Verification items for the finished model (mm, model axes). Face numbers are marked on the shaded views. A direction names the side the tool comes from. Coordinates: 2 decimals unless noted, no trailing zeros. Write each loop counter-clockwise with the first axis right and the second up, starting at its lowest first coordinate (ties: lowest second). Pieces come first, ordered by that corner, then holes. Notation, with made-up numbers: (-2.5, 65.5) -> (47.5, 65.5) arc R21 cw to (47.5, 90.5) -> close; hole circle Ø8 at (87.5, 44.5). An arc over 180 degrees is marked (long way). Write item = value, one per line. Start each with the question number.
(1) Set-up check for the marked faces 1, 2 and 3: record each of +Z, -Z, +X, -X, +Y, -Y from which the full face is reachable in a straight line by a thin tool's end or side.
(2) Material ranges on probe 1 along Z at (x, y) = (16, 57); probe 2 along Y at (x, z) = (-27, -1); probe 3 along X at (y, z) = (105, -10.5), recorded low to high. Write a range as [from, to].
(3) Section check A-A (y = 48.5). Record the cut outline in (x, z).
(4) Section check C-C (z = 8). Record the cut outline in (x, y), plus the area to 3 significant figures.
(5) Gauge pin test, flat ends, axial feed: pin 1 Ø10.5 at (y, z) = (132, 5.5) entering from -X; pin 2 Ø6 at (y, z) = (34, -28.5) entering from -X; pin 3 Ø4 at (y, z) = (58, -33) entering from +X. Record the tip position at first contact, or that the pin passes through.
(6) Section check B-B (x = -8). Record the cut outline in (y, z), plus the area to 3 significant figures.
(7) Section check D-D (y = 134.5). Record the cut outline in (x, z).
```python
from build123d import *

# Parameters (mm, degrees)
EXTRUDE_1_DEPTH     = 170
SKETCH_3_W          = 66.248134628
SKETCH_3_H          = 139.711623237
CUT_EXTRUDE_1_DEPTH = 170


with BuildPart() as part:
    # 草图1 → 凸台-拉伸1 (new body)
    with BuildSketch(Plane(origin=(0, 0, 0), x_dir=(1, 0, 0), z_dir=(0, 1, 0))):
        with BuildLine():
            Line((-25.11018553, 16.026132479), (38.850953275, 16.026132479))
            Line((38.850953275, 16.026132479), (38.850953275, -18.973867521))
            Line((38.850953275, -18.973867521), (-64.562961279, -18.973867521))
            ThreePointArc((-64.562961279, -18.973867521), (-81.696259365, 35.906986737), (-25.11018553, 46.079219305))
            Line((-25.11018553, 46.079219305), (-25.11018553, 16.026132479))
        make_face()
    extrude(amount=EXTRUDE_1_DEPTH)

    # 草图3 → 切除-拉伸1 (cut)
    with BuildSketch(Plane.XY.offset(18.973867521)):
        with Locations((-54.667445772, 132.083845768)):
            Rectangle(SKETCH_3_W, SKETCH_3_H)
    extrude(amount=-CUT_EXTRUDE_1_DEPTH, mode=Mode.SUBTRACT)


solid = part.part
```
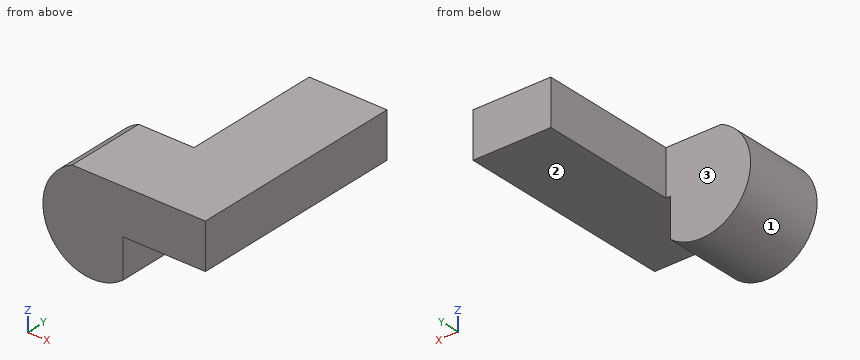
Response:
q1.face_1 = +Y, -Y
q1.face_2 = -Z, +X, +Y, -Y
q1.face_3 = +Z, -Z, -X, +Y
q2.probe_1 = [-16.03, 18.97]
q2.probe_2 = [0, 62.23]
q2.probe_3 = [-21.54, 38.85]
q3.outline = (-64.56, 18.97) arc R38.34 ccw (long way) to (-25.11, -46.08) -> (-25.11, -16.03) -> (38.85, -16.03) -> (38.85, 18.97) -> close
q4.outline = (-78.79, 0) -> (38.85, 0) -> (38.85, 170) -> (-21.54, 170) -> (-21.54, 62.23) -> (-78.79, 62.23) -> close
q4.area = 13,800 mm2
q5.pin_1 = -21.54
q5.pin_2 = -86.06
q5.pin_3 = -25.11
q6.outline = (0, -16.03) -> (170, -16.03) -> (170, 18.97) -> (0, 18.97) -> close
q6.area = 5,950 mm2
q7.outline = (-21.54, -16.03) -> (38.85, -16.03) -> (38.85, 18.97) -> (-21.54, 18.97) -> close
